Input: part model. Units: mm. Frame: model coordinates. A direction names the side the tool comes from. Round coordinates to 2 decimals unless told otherwise and drop trailing zeros. Loops run counter-clockwise (first coordinate to the right, second up) from the corner with the lowest first, then second, coordinate; pieces in that order, holes last. Notation, with made-up numbers: (9.5, 56) -> (53.5, 56) arc R13 ccw to (53.5, 62) -> close; hole circle Ø6 at (-33, 80). An arc over 180 degrees is marked (long way). Answer as a JSON object with one key per item and string values.
```python
from build123d import *

# Parameters (mm, degrees)
SKETCH1_W           = 60
SKETCH1_H           = 60
BOSS_EXTRUDE1_DEPTH = 80
SKETCH2_W           = 40
SKETCH2_H           = 40
CUT_EXTRUDE1_DEPTH  = 20
SKETCH3_W           = 20
SKETCH3_H           = 20
CUT_EXTRUDE2_DEPTH  = 136
BOSS_EXTRUDE2_DEPTH = 40
CUT_EXTRUDE3_DEPTH  = 10
SKETCH7_W           = 40
SKETCH7_H           = 40
CUT_EXTRUDE4_DEPTH  = 20
SKETCH8_W           = 20
SKETCH8_H           = 20
CUT_EXTRUDE5_DEPTH  = 20
BOSS_EXTRUDE3_DEPTH = 40
CUT_EXTRUDE6_DEPTH  = 10
SKETCH11_W          = 40
SKETCH11_H          = 40
CUT_EXTRUDE7_DEPTH  = 20
SKETCH12_W          = 20
SKETCH12_H          = 20
CUT_EXTRUDE8_DEPTH  = 20


with BuildPart() as part:
    # Sketch1 → Boss-Extrude1 (new body)
    with BuildSketch(Plane.XY):
        with Locations((30, 30)):
            Rectangle(SKETCH1_W, SKETCH1_H)
    extrude(amount=BOSS_EXTRUDE1_DEPTH)

    # Sketch2 → Cut-Extrude1 (cut)
    with BuildSketch(Plane.XY.offset(80)):
        with Locations((30, 30)):
            Rectangle(SKETCH2_W, SKETCH2_H)
    extrude(amount=-CUT_EXTRUDE1_DEPTH, mode=Mode.SUBTRACT)

    # Sketch3 → Cut-Extrude2 (cut)
    with BuildSketch(Plane.XY.offset(60)):
        with Locations((30, 30)):
            Rectangle(SKETCH3_W, SKETCH3_H)
    extrude(amount=-CUT_EXTRUDE2_DEPTH, mode=Mode.SUBTRACT)

    # Sketch5 → Boss-Extrude2 (add)
    with BuildSketch(Plane(origin=(0, 0, 0), x_dir=(-1, 0, 0), z_dir=(0, 0, -1))):
        Polygon((10, 80), (-10, 60), (0, 60), (0, 0), (-10, 0), (10, -20), (30, -20), (50, 0), (50, 60), (30, 80), align=None)
    extrude(amount=-BOSS_EXTRUDE2_DEPTH)

    # Sketch6 → Cut-Extrude3 (cut)
    with BuildSketch(Plane.XY.offset(40)):
        Polygon((-40, 70), (0, 70), (-10, 80), (-30, 80), align=None)
        Polygon((0, -10), (-40, -10), (-30, -20), (-10, -20), align=None)
    extrude(amount=-CUT_EXTRUDE3_DEPTH, mode=Mode.SUBTRACT)

    # Sketch7 → Cut-Extrude4 (cut)
    with BuildSketch(Plane.XY.offset(40)):
        with Locations((-30, 30)):
            Rectangle(SKETCH7_W, SKETCH7_H)
    extrude(amount=-CUT_EXTRUDE4_DEPTH, mode=Mode.SUBTRACT)

    # Sketch8 → Cut-Extrude5 (cut)
    with BuildSketch(Plane.XY.offset(20)):
        with Locations((-30, 30)):
            Rectangle(SKETCH8_W, SKETCH8_H)
    extrude(amount=-CUT_EXTRUDE5_DEPTH, mode=Mode.SUBTRACT)

    # Sketch9 → Boss-Extrude3 (add)
    with BuildSketch(Plane(origin=(0, 0, 0), x_dir=(-1, 0, 0), z_dir=(0, 0, -1))):
        Polygon((-50, 60), (-70, 80), (-90, 80), (-110, 60), (-110, 0), (-90, -20), (-70, -20), (-50, 0), (-60, 0), (-60, 60), align=None)
    extrude(amount=-BOSS_EXTRUDE3_DEPTH)

    # Sketch10 → Cut-Extrude6 (cut)
    with BuildSketch(Plane.XY.offset(40)):
        Polygon((60, 70), (100, 70), (90, 80), (70, 80), align=None)
        Polygon((60, -10), (100, -10), (90, -20), (70, -20), align=None)
    extrude(amount=-CUT_EXTRUDE6_DEPTH, mode=Mode.SUBTRACT)

    # Sketch11 → Cut-Extrude7 (cut)
    with BuildSketch(Plane.XY.offset(40)):
        with Locations((90, 30)):
            Rectangle(SKETCH11_W, SKETCH11_H)
    extrude(amount=-CUT_EXTRUDE7_DEPTH, mode=Mode.SUBTRACT)

    # Sketch12 → Cut-Extrude8 (cut)
    with BuildSketch(Plane.XY.offset(20)):
        with Locations((90, 30)):
            Rectangle(SKETCH12_W, SKETCH12_H)
    extrude(amount=-CUT_EXTRUDE8_DEPTH, mode=Mode.SUBTRACT)


solid = part.part
```
1) Section C-C, the plane x = 98. Output: boundary loops of the cut face in (y, z), plus the area to 3 significant figures.
Output:
{"outline": "(-12, 0) -> (20, 0) -> (20, 20) -> (10, 20) -> (10, 40) -> (-10, 40) -> (-10, 30) -> (-12, 30) -> close; (40, 0) -> (72, 0) -> (72, 30) -> (70, 30) -> (70, 40) -> (50, 40) -> (50, 20) -> (40, 20) -> close", "area": "2,120 mm^2"}
2) Reachability of faces 5 (the face through (40, 30, 30)), 6 (the face through (80, -10, 35)), 7 (the face through (-20, 70, 35)), 8 (the face through (-30, 50, 30)) from +Z, -Z, +X, -X, +Y, -Y: full face, straight path, thin tool, end or side. Return the list, or none.
Output:
{"face 5": "+Z, -Z", "face 6": "+Z, +X, -X, -Y", "face 7": "+Z, +X, -X, +Y", "face 8": "+Z, -X"}
3) Section B-B, the plane z = 74. Output: boundary loops of the cut face in (x, y).
Output:
{"outline": "(0, 0) -> (60, 0) -> (60, 60) -> (0, 60) -> close; hole (10, 10) -> (50, 10) -> (50, 50) -> (10, 50) -> close"}
4) Contact query for flat-ended pins moving along their axis: P1, Ø10, axis at x = 97.5, z = 28, coming from the -Y side; P2, Ø5, axis at x = 86.5, z = 34, coming from the +Y side; P3, Ø3, axis at x = -11.5, y = -16, coming from the +Z side. Output: stop coordinate, or through.
Output:
{"P1": "stops at y = -17.5", "P2": "stops at y = 70", "P3": "stops at z = 30"}
5) Section A-A, the plane y = -7.5. Output: boundary loops of the cut face in (x, z).
Output:
{"outline": "(-42.5, 0) -> (2.5, 0) -> (2.5, 40) -> (-42.5, 40) -> close; (57.5, 0) -> (102.5, 0) -> (102.5, 40) -> (57.5, 40) -> close"}
6) Section D-D, the plane y = 32. Output: boundary loops of the cut face in (x, z).
Output:
{"outline": "(-50, 0) -> (-40, 0) -> (-40, 20) -> (-50, 20) -> close; (-20, 0) -> (20, 0) -> (20, 60) -> (10, 60) -> (10, 80) -> (0, 80) -> (0, 40) -> (-10, 40) -> (-10, 20) -> (-20, 20) -> close; (40, 0) -> (80, 0) -> (80, 20) -> (70, 20) -> (70, 40) -> (60, 40) -> (60, 80) -> (50, 80) -> (50, 60) -> (40, 60) -> close; (100, 0) -> (110, 0) -> (110, 20) -> (100, 20) -> close"}
7) Draft query along X for faces 1 (the face through (31.1, 19.6, 0)), 2 (the face through (70, 30, 30)), 3 (the face through (100, 30, 10)), 4 (the face through (0, 30, 60)). Return one class per face: +X half, -X half, draft (parallel to the pull), parting line (faces both ways), or undercut.
Output:
{"face 1": "draft", "face 2": "+X half", "face 3": "undercut", "face 4": "-X half"}
8) Ray query, probe 1 along X at (y, z) = (35.5, 56.5); probe 2 along X at (y, z) = (32, 72.5). Return the intervals inside material, ascending.
Output:
{"probe 1": "x = 0 to 20, 40 to 60", "probe 2": "x = 0 to 10, 50 to 60"}
